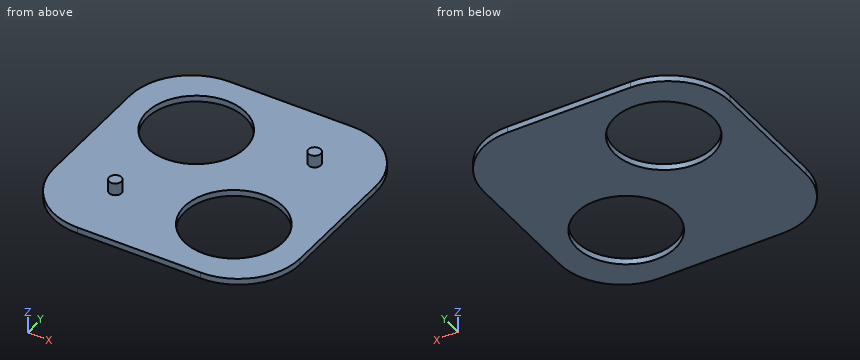
```python
from build123d import *

# Parameters (mm, degrees)
BOSS_EXTRUDE1_DEPTH = 50
SKETCH2_R           = 50
BOSS_EXTRUDE2_DEPTH = 100
SKETCH3_R           = 400
CUT_EXTRUDE1_DEPTH  = 100


with BuildPart() as part:
    # Sketch1 → Boss-Extrude1 (new body)
    with BuildSketch(Plane.XY):
        with BuildLine():
            Line((-500, 1000), (500, 1000))
            ThreePointArc((500, 1000), (853.553390593, 853.553390593), (1000, 500))
            Line((1000, 500), (1000, -500))
            ThreePointArc((1000, -500), (853.553390593, -853.553390593), (500, -1000))
            Line((500, -1000), (-500, -1000))
            ThreePointArc((-500, -1000), (-853.553390593, -853.553390593), (-1000, -500))
            Line((-1000, -500), (-1000, 500))
            ThreePointArc((-1000, 500), (-853.553390593, 853.553390593), (-500, 1000))
        make_face()
    extrude(amount=BOSS_EXTRUDE1_DEPTH)

    # Sketch2 → Boss-Extrude2 (add)
    with BuildSketch(Plane.XY.offset(50)):
        with Locations(Location((-500, -500, 0), (0, 0, 180))):
            Circle(SKETCH2_R)
        with Locations(Location((500, 500, 0), (0, 0, 180))):
            Circle(SKETCH2_R)
    extrude(amount=BOSS_EXTRUDE2_DEPTH)

    # Sketch3 → Cut-Extrude1 (cut)
    with BuildSketch(Plane.XY.offset(50)):
        with Locations((400, -400)):
            Circle(SKETCH3_R)
        with Locations((-400, 400)):
            Circle(SKETCH3_R)
    extrude(amount=-CUT_EXTRUDE1_DEPTH, mode=Mode.SUBTRACT)


solid = part.part
```
The listing builds one solid part. Answer for the finished solid, in the listing's coordinates (mm). Coordinates: 2 decimals unless noted, no trailing zeros. Write each loop counter-clockwise with the first axis right and the second up, starting at its lowest first coordinate (ties: lowest second). Pieces come first, ordered by that corner, then holes. Notation, with made-up numbers: M 1.5,89 L 56.5,89 A17 ccw 56.5,115 Z; hole C 32.25,-21.75 d6. An arc over 180 degrees is marked long. Use a Markdown table: item, result. Add a question column.
1. Section C-C (z = 101.5) is taken. Give the vertices of the cut face in (x, y), plus the area to 3 significant figures.
2. Section A-A (y = 400) is taken. Give the vertices of the cut face in (x, z), plus the area to 3 significant figures.
3. Given P1, Ø10, axis at y = 789, z = 43.5, coming from the +X side; P2, Ø4, axis at y = -549, z = 28, coming from the +X side, each flat-ended and moving along its own axis, determine where each tip first touches the part or whether it passes through.
4. Section D-D (y = -877) is taken. Give the vertices of the cut face in (x, z).
5. Straight lines are drawn through the part: line 1 along Y through (x, z) = (400, 23); line 2 along Y through (x, z) = (-400, 39); line 3 along Z through (x, y) = (-912, 136.5). For each, find the intervals that lie inside material, in ascending order. Write a range as [from, to].
Data:
| question | item | result |
|---|---|---|
| 1 | outline | C -500,-500 d100; C 500,500 d100 |
| 1 | area | 15,700 mm2 |
| 2 | outline | M -1000,0 L -800,0 L -800,50 L -1000,50 Z; M 0,0 L 1000,0 L 1000,50 L 0,50 Z |
| 2 | area | 60,000 mm2 |
| 3 | P1 | stops at x = 911.51 |
| 3 | P2 | stops at x = 997.79 |
| 4 | outline | M -828.44,0 L 828.44,0 L 828.44,50 L -828.44,50 Z |
| 5 | line 1 | y = [-1000, -800], [0, 1000] |
| 5 | line 2 | y = [-1000, 0], [800, 1000] |
| 5 | line 3 | z = [0, 50] |
